from build123d import *

# Parameters (mm, degrees)
EXTRUDE_1_DEPTH     = 14
SKETCH_2_R          = 1.3
CUT_EXTRUDE_1_DEPTH = 35.365680555
SKETCH_4_W          = 6
SKETCH_4_H          = 11
CUT_EXTRUDE_3_DEPTH = 34.526109228


with BuildPart() as part:
    # 草圖1 → 填料-伸長1 (new body)
    with BuildSketch(Plane(origin=(0, 0, 0), x_dir=(0, 0, -1), z_dir=(1, 0, 0))):
        Polygon((0, 0), (12, 0), (12, 1), (1, 1), (1, 29), (0, 29), align=None)
    extrude(amount=EXTRUDE_1_DEPTH)

    # 草圖2 → 除料-伸長1 (cut, through all)
    with BuildSketch(Plane.XY):
        with Locations((4, 26)):
            Circle(SKETCH_2_R)
        with Locations((4, 18)):
            Circle(SKETCH_2_R)
    extrude(amount=-CUT_EXTRUDE_1_DEPTH, mode=Mode.SUBTRACT)

    # 草圖4 → 除料-伸長3 (cut, through all)
    with BuildSketch(Plane(origin=(0, 1, 0), x_dir=(1, 0, 0), z_dir=(0, 1, 0))):
        with Locations((3, 6.5)):
            Rectangle(SKETCH_4_W, SKETCH_4_H)
    extrude(amount=-CUT_EXTRUDE_3_DEPTH, mode=Mode.SUBTRACT)


solid = part.part
Geometry: final body of the model. Coordinates: model frame, mm. A direction names the side the tool comes from. Round coordinates to 2 decimals unless told otherwise and drop trailing zeros. Loops run counter-clockwise (first coordinate to the right, second up) from the corner with the lowest first, then second, coordinate; pieces in that order, holes last.
Q1. Access query for faces 1 (the flat face through (6, 0.5, -6.4)), 2 (the flat face through (7, 15, 0)), 3 (the flat face through (10, 1, -7)). Directions: +Z, -Z, +X, -X, +Y, -Y. A direction counts if a zero-diameter tool reaches every point of the face in a straight line with its end or side. Return the directions, or none.
Q2. Material intervals for L1, parallel to Y at x = 4, z = -0.3; L2, parallel to Y at x = 6.5, z = -1.75; L3, parallel to Z at x = 12.75, y = 14, sorted ascending.
Q3. Pull-direction query (X, two-part tool) for faces 4 (the flat face through (0, 14.7, -0.5)), 5 (the flat face through (6.9, 29, -0.5)), 6 (the cylindrical face through (3.72, 16.73, -0.49)), 7 (the cylindrical face through (3.72, 24.73, -0.49)); classes: released by +X, released by -X, zero draft, split by the parting line, or undercut.
Q4. Section C-C on y = 26.5. Return loops of the section in (x, z).
Q5. Section B-B on y = 18. Return loops of the section in (x, z).
Q6. Pin query (flat end, axial travel): P1, Ø3, axis at x = 4, y = 18, coming from the +Z side; P2, Ø1.5, axis at x = 2, y = 21, coming from the -Z side. Return the tip coordinate at first contact, or that it passes through.
Q7. Section A-A on x = 4. Return loops of the section in (y, z).
Q8. Section D-D on x = 8. Return loops of the section in (y, z).
Evaluation:
1. face 1: -Z, -X, +Y, -Y
1. face 2: +Z, +X, -X, +Y, -Y
1. face 3: -Z, +X, -X, +Y
2. L1: y = 0 to 16.7, 19.3 to 24.7, 27.3 to 29
2. L2: y = 0 to 1
2. L3: z = -1 to 0
3. face 4: released by -X
3. face 5: zero draft
3. face 6: undercut
3. face 7: undercut
4. outline: (0, -1) - (2.8, -1) - (2.8, 0) - (0, 0) - close; (5.2, -1) - (14, -1) - (14, 0) - (5.2, 0) - close
5. outline: (0, -1) - (2.7, -1) - (2.7, 0) - (0, 0) - close; (5.3, -1) - (14, -1) - (14, 0) - (5.3, 0) - close
6. P1: stops at z = 0
6. P2: stops at z = -1
7. outline: (0, -1) - (16.7, -1) - (16.7, 0) - (0, 0) - close; (19.3, -1) - (24.7, -1) - (24.7, 0) - (19.3, 0) - close; (27.3, -1) - (29, -1) - (29, 0) - (27.3, 0) - close
8. outline: (0, -12) - (1, -12) - (1, -1) - (29, -1) - (29, 0) - (0, 0) - close
